Model file for the job. Use its own axes, mm. A direction names the side the tool comes from. Coordinates: 2 decimals unless noted, no trailing zeros. Write each loop counter-clockwise with the first axis right and the second up, starting at its lowest first coordinate (ties: lowest second). Pieces come first, ordered by that corner, then holes. Notation, with made-up numbers: (-10, 52.25) - (33, 52.25) arc R29 cw to (33, 77.25) - close; hole circle Ø9 at (-6.5, -37). An arc over 180 degrees is marked (long way). Put each result on its own line as item: value. Start each with the question number.
1. Saw through at B-B, the plane z = -152.4. Write the cut outline in (x, y).
2. Drop flat-ended pins along their axis: P1, Ø4.5, axis at y = -19.05, z = 92.075, coming from the -X side; P2, Ø9, axis at y = 50.8, z = -92.075, coming from the +X side. Give the stop position or say it passes through.
3. Drill centre lines: L1, parallel to Z at x = 2, y = 50.8; L2, parallel to Y at x = 5, z = -152.4; L3, parallel to Z at x = 1.5, y = 5.5. Where is each one in solid material? Low to high. Write a range as from..to.
4. Which spindle directions (+Z, -Z, +X, -X, +Y, -Y) get a long thin tool onto all of the face, cutting with end or side? Do faces 4 (the face through (3, -38.1, 1)), 5 (the face through (3, -63.5, -145)). Say none if no direction does.
5. Pull direction Z, two halves, no side cores. Call faces 1 (the face through (3.219, 10.403, -165.598)), 2 (the face through (3, -63.5, 147)), 3 (the face through (3, -1, 196.85)): released by +Z, released by -Z, zero draft, split by the parting line, or undercut.
6. Saw through at A-A, the plane z = 0. Write the cut outline in (x, y), plus the area to 3 significant figures.
7. Saw through at D-D, the plane x = 1.75. Give the number of separate pieces and of enclosed holes in the cut face, plus the area to 3 significant figures.
8. Saw through at C-C, the plane y = 25. Write the cut outline in (x, z).
```python
from build123d import *

# Parameters (mm, degrees)
SKETCH1_W                                          = 393.7
SKETCH1_H                                          = 127
BOSS_EXTRUDE1_DEPTH                                = 6.35
SKETCH2_R                                          = 14.2875
CUT_EXTRUDE1_DEPTH                                 = 207.935968357
F_10_CLEARANCE_HOLE1_D                             = 4.9784
CSK_FOR_10_FLAT_HEAD_MACHINE_SCREW_100_D           = 5.6134
CSK_FOR_10_FLAT_HEAD_MACHINE_SCREW_100_CSINK_D     = 9.779
CSK_FOR_10_FLAT_HEAD_MACHINE_SCREW_100_CSINK_ANGLE = 100
SKETCH23_W                                         = 190.5
SKETCH23_H                                         = 25.4
CUT_EXTRUDE6_DEPTH                                 = 207.935968357


with BuildPart() as part:
    # Sketch1 → Boss-Extrude1 (new body)
    with BuildSketch(Plane(origin=(0, 0, 0), x_dir=(0, 0, -1), z_dir=(1, 0, 0))):
        Rectangle(SKETCH1_W, SKETCH1_H)
    extrude(amount=BOSS_EXTRUDE1_DEPTH)

    # Sketch2 → Cut-Extrude1 (cut, through all)
    with BuildSketch(Plane(origin=(6.35, 0, 0), x_dir=(0, 0, -1), z_dir=(1, 0, 0))):
        with Locations((0, 15.875)):
            Circle(SKETCH2_R)
        with Locations((-152.4, 15.875)):
            Circle(SKETCH2_R)
        with Locations((152.4, 15.875)):
            Circle(SKETCH2_R)
        with Locations((-152.4, -44.45)):
            Circle(SKETCH2_R)
        with Locations((152.4, -44.45)):
            Circle(SKETCH2_R)
    extrude(amount=-CUT_EXTRUDE1_DEPTH, mode=Mode.SUBTRACT)

    # #10 Clearance Hole1 (through all)
    with Locations(Plane(origin=(6.35, 0, 0), x_dir=(0, 0, -1), z_dir=(1, 0, 0))):
        with Locations((-190.754, 19.05), (-190.754, -19.05), (190.754, 19.05), (190.754, -19.05)):
            Hole(F_10_CLEARANCE_HOLE1_D / 2)

    # CSK for #10 Flat Head Machine Screw (100)1 (through all)
    with Locations(Plane(origin=(6.35, 0, 0), x_dir=(0, 0, -1), z_dir=(1, 0, 0))):
        with Locations((-92.075, 50.8), (92.075, 50.8), (-92.075, -19.05), (92.075, -19.05)):
            CounterSinkHole(CSK_FOR_10_FLAT_HEAD_MACHINE_SCREW_100_D / 2, CSK_FOR_10_FLAT_HEAD_MACHINE_SCREW_100_CSINK_D / 2, counter_sink_angle=CSK_FOR_10_FLAT_HEAD_MACHINE_SCREW_100_CSINK_ANGLE)

    # Sketch23 → Cut-Extrude6 (cut, through all)
    with BuildSketch(Plane(origin=(6.35, 0, 0), x_dir=(0, 0, -1), z_dir=(1, 0, 0))):
        with Locations((0, -50.8)):
            Rectangle(SKETCH23_W, SKETCH23_H)
    extrude(amount=-CUT_EXTRUDE6_DEPTH, mode=Mode.SUBTRACT)


solid = part.part
```
Final values:
1. outline: (0, -63.5) - (6.35, -63.5) - (6.35, -58.74) - (0, -58.74) - close; (0, -30.16) - (6.35, -30.16) - (6.35, 1.59) - (0, 1.59) - close; (0, 30.16) - (6.35, 30.16) - (6.35, 63.5) - (0, 63.5) - close
2. P1: passes through
2. P2: stops at x = 6.02
3. L1: z = -196.85..-94.88, -89.27..89.27, 94.88..196.85
3. L2: y = -63.5..-58.74, -30.16..1.59, 30.16..63.5
3. L3: z = -196.85..-162.22, -142.58..-9.82, 9.82..142.58, 162.22..196.85
4. face 4: +X, -X, -Y
4. face 5: +Z, -Z, +X, -X, -Y
5. face 1: undercut
5. face 2: zero draft
5. face 3: released by +Z
6. outline: (0, -38.1) - (6.35, -38.1) - (6.35, 1.59) - (0, 1.59) - close; (0, 30.16) - (6.35, 30.16) - (6.35, 63.5) - (0, 63.5) - close
6. area: 464 mm²
7. separate pieces: 1
7. enclosed holes: 13
7. area: 41,800 mm²
8. outline: (0, -196.85) - (6.35, -196.85) - (6.35, -163.39) - (0, -163.39) - close; (0, -141.41) - (6.35, -141.41) - (6.35, -10.99) - (0, -10.99) - close; (0, 10.99) - (6.35, 10.99) - (6.35, 141.41) - (0, 141.41) - close; (0, 163.39) - (6.35, 163.39) - (6.35, 196.85) - (0, 196.85) - close
